Can you work these out from the model? Positions are in its coordinate system, mm. Face numbers are marked on the shaded views. A direction names the side the tool comes from. Give positions to 0.01 mm unless a question says otherwise; leave off trailing zeros. Loops run counter-clockwise (first coordinate to the right, second up) from the corner with the lowest first, then second, coordinate; pieces in that order, holes last. Notation, with made-up numbers: (83, 46) - (111, 46) arc R16 cw to (111, 66) - close; hole circle Ø9 at (32.5, -2). An arc over 180 degrees is marked (long way). Answer as a JSON object with one key per item and string values.
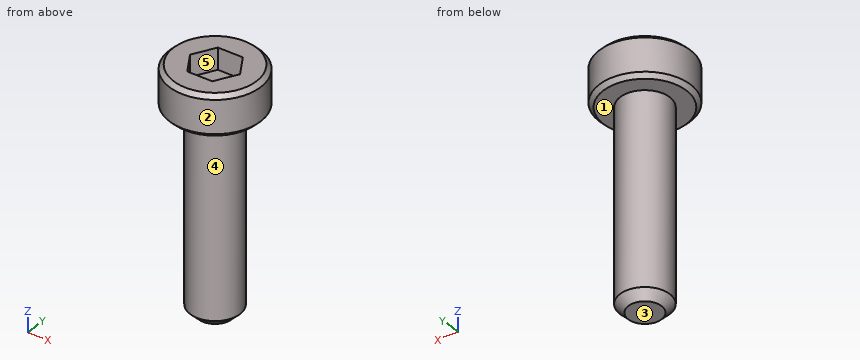
```python
from build123d import *

# Parameters (mm, degrees)
F0_R     = 1.5
F1_DEPTH = 12
F2_SIZE  = 0.5
F0_R_2   = 2.75
F3_DEPTH = 2.5
F4_SIZE  = 0.25
F6_DEPTH = 1.3


with BuildPart() as f1:
    # F0 (on Top) → F1 (new body)
    with BuildSketch(Plane.XY):
        Circle(F0_R)
    extrude(amount=-F1_DEPTH)

    # F2
    f2_edges = [f1.edges().sort_by_distance(p)[0] for p in [
        (-1.5, 0, -12),
    ]]
    chamfer(f2_edges, length=F2_SIZE)

    # F0 (on Top) → F3 (join)
    with BuildSketch(Plane.XY):
        Circle(F0_R_2)
        Circle(F0_R, mode=Mode.SUBTRACT)
        Circle(F0_R)
    extrude(amount=F3_DEPTH)

    # F4
    f4_edges = [f1.edges().sort_by_distance(p)[0] for p in [
        (-2.75, 0, 2.5),
        (-2.75, 0, 0),
    ]]
    chamfer(f4_edges, length=F4_SIZE)

    # F5 (on face) → F6 (cut)
    with BuildSketch(Plane.XY.offset(2.5)):
        Polygon((0.75963, -1.281313), (1.489464, 0.017202), (0.729835, 1.298515), (-0.75963, 1.281313), (-1.489464, -0.017202), (-0.729835, -1.298515), align=None)
    extrude(amount=-F6_DEPTH, mode=Mode.SUBTRACT)


solid = f1.part
```
1) Which directions (+Z, -Z, +X, -X, +Y, -Y) give clear straight access to the entire face, cutting with the end or side of a thin tool? Please do the marked faces 1 and 2.
Check sheet entries:
{"face 1": "-Z", "face 2": "+Z, -Z"}
2) Imagine slicing it at B-B on x = 0. Write out the boundary of the cut face in (y, z).
Check sheet entries:
{"outline": "(-2.75, 0.25) - (-2.5, 0) - (-1.5, 0) - (-1.5, -11.5) - (-1, -12) - (1, -12) - (1.5, -11.5) - (1.5, 0) - (2.5, 0) - (2.75, 0.25) - (2.75, 2.25) - (2.5, 2.5) - (1.29, 2.5) - (1.29, 1.2) - (-1.29, 1.2) - (-1.29, 2.5) - (-2.5, 2.5) - (-2.75, 2.25) - close"}
3) Imagine slicing it at A-A on z = -9.5. Write out the boundary of the cut face in (x, y).
Check sheet entries:
{"outline": "circle Ø3 at (0, 0)"}
4) I'm going to push flat-ended pins straight in: P1, Ø1.5, axis at x = -0.5, z = -8, coming from the -Y side; P2, Ø3, axis at x = -2, z = -8, coming from the -Y side; P3, Ø1.5, axis at y = -2, z = -4.5, coming from the +X side. Where does each tip first touch, or does it pass through?
Check sheet entries:
{"P1": "y = -1.5", "P2": "y = -1.41", "P3": "x = 0.83"}
5) I need wall thicknesses on L1, parallel to Z at x = -1.45, y = -1.8; L2, parallel to Z at x = -0.5, y = 0.1; L3, parallel to X at y = -0.2, z = -8. Which ranges of each line are inside material? Lowest first, please.
Check sheet entries:
{"L1": "0 to 2.5", "L2": "-12 to 1.2", "L3": "-1.49 to 1.49"}
6) If we mould it in two halves opening along X, with no side actions, what happens to the marked faces 3, 4 and 5? For each: released by +X, released by -X, zero draft, split by the parting line, or undercut.
Check sheet entries:
{"face 3": "zero draft", "face 4": "split by the parting line", "face 5": "undercut"}
